Autodesk Fusion 360 part; units mm, degrees
sketch "Sketch1" plane through (0, 0, 0) normal (0, 0, 1) x (1, 0, 0)
  line L0 (9, 9) -> (-9, 9)
  line L1 (-9, 9) -> (-9, -9)
  line L2 (-9, -9) -> (9, -9)
  line L3 (9, -9) -> (9, 9)
  line L4 (9, 9) -> (-9, -9) construction
  line L5 (-9, 9) -> (9, -9) construction
  dimension "d1" = 18
  dimension "d2" = 18
extrude "Extrude1" add sketch "Sketch1" along normal blind 3
sketch "Sketch3" plane through (0, 0, 0) normal (0, 1, 0) x (1, 0, 0)
  circle A0 centre (0, -4) radius 3
  circle A1 centre (0, -4) radius 2
  dimension "d5" = 6
  dimension "d6" = 4
extrude "Extrude2" add sketch "Sketch3" along normal mid plane 3
Could you check a few things on this model? Use its own coordinates, in mm. A direction names the side the tool comes from. Coordinates: 2 decimals unless noted, no trailing zeros. Order: outer loops, then holes, each group sorted by start corner. A loop starts at its lowest first (then second) coordinate and runs counter-clockwise, first axis right, second up.
Q1. Suppose I cut it at C-C on y = -7. Please give me the cut outline in (x, z), and give its area (3 significant figures).
Q2. Suppose I cut it at A-A on x = 0. Please give me the cut outline in (y, z).
Q3. Thinking about a two-plate mould opening in Z: for faces 3 (the flat face through (0, 0, 0)), 4 (the flat face through (0, 1.5, 6.3)), 5 (the cylindrical face through (0, 0, 6)), which applies, released by +Z, released by -Z, zero draft, split by the parting line, or undercut?
Q4. Will these pins go through, and if not, where does the flat tip stop? pin 1 (2 mm diameter, centred on x = 6.5, y = 1.5, fed in from +Z); pin 2 (3 mm diameter, centred on x = 0, z = 5, fed in from -Y); pin 3 (1 mm diameter, centred on y = 0, z = 4.5, fed in from +X).
Q5. Suppose I cut it at B-B on z = 4. Please give me the cut outline in (x, y).
Q6. Which directions (+Z, -Z, +X, -X, +Y, -Y) give clear straight access to the entire face, cutting with the end or side of a thin tool? Please do faces 1 (the flat face through (0, -1.5, 6.3)), 2 (the flat face through (0, -9, 1)).
Q7. Please list where these lines run through material, in increasing order: L1, parallel to Z at x = 0, y = -0.3; L2, parallel to X at y = -0.1, z = 4; L3, parallel to Z at x = 1, y = -3.5.
Answer:
1. outline: (-9, 0) - (9, 0) - (9, 3) - (-9, 3) - close
1. area: 54.0 mm2
2. outline: (-9, 0) - (9, 0) - (9, 3) - (-9, 3) - close; (-1.5, 6) - (1.5, 6) - (1.5, 7) - (-1.5, 7) - close
3. face 3: released by -Z
3. face 4: zero draft
3. face 5: undercut
4. pin 1: stops at z = 3
4. pin 2: stops at y = -1.5
4. pin 3: stops at x = 3
5. outline: (-3, -1.5) - (-2, -1.5) - (-2, 1.5) - (-3, 1.5) - close; (2, -1.5) - (3, -1.5) - (3, 1.5) - (2, 1.5) - close
6. face 1: +Z, +X, -X, -Y
6. face 2: +Z, -Z, +X, -X, -Y
7. L1: z = 0 to 3, 6 to 7
7. L2: x = -3 to -2, 2 to 3
7. L3: z = 0 to 3
